Part model, mm, in its own coordinate system. Face numbers are marked on the shaded views. Round coordinates to 2 decimals unless told otherwise and drop trailing zeros. Order: outer loops, then holes, each group sorted by start corner. A loop starts at its lowest first (then second) coordinate and runs counter-clockwise, first axis right, second up. Notation, with made-up numbers: M 28,56 L 60,56 A15 cw 60,77 Z; hole C 25,44.25 d4. An arc over 180 degrees is marked long. One line per question, with ' | ' between items.
from build123d import *

# Parameters (mm, degrees)
F0_R           = 5.5
F1_DEPTH       = 18
F2_R           = 1
F3_R           = 4.375
F4_DEPTH       = 7.5
F5_SIZE        = 1
F7_D           = 5
F7_CSINK_D     = 9
F7_CSINK_ANGLE = 90


with BuildPart() as f1:
    # F0 (on Front) → F1 (new body)
    with BuildSketch(Plane.XZ):
        Circle(F0_R)
    extrude(amount=F1_DEPTH)

    # F2
    f2_edges = [f1.edges().sort_by_distance(p)[0] for p in [
        (-5.5, -18, 0),
    ]]
    fillet(f2_edges, radius=F2_R)

    # F3 (on face) → F4 (join)
    with BuildSketch(Plane(origin=(0, 0, 0), x_dir=(-1, 0, 0), z_dir=(0, 1, 0))):
        Circle(F3_R)
    extrude(amount=F4_DEPTH)

    # F5
    f5_edges = [f1.edges().sort_by_distance(p)[0] for p in [
        (4.375, 7.5, 0),
    ]]
    chamfer(f5_edges, length=F5_SIZE)

    # F7 (through all)
    with Locations(Plane.XZ.offset(18)):
        with Locations((0, 0)):
            CounterSinkHole(F7_D / 2, F7_CSINK_D / 2, counter_sink_angle=F7_CSINK_ANGLE)


solid = f1.part
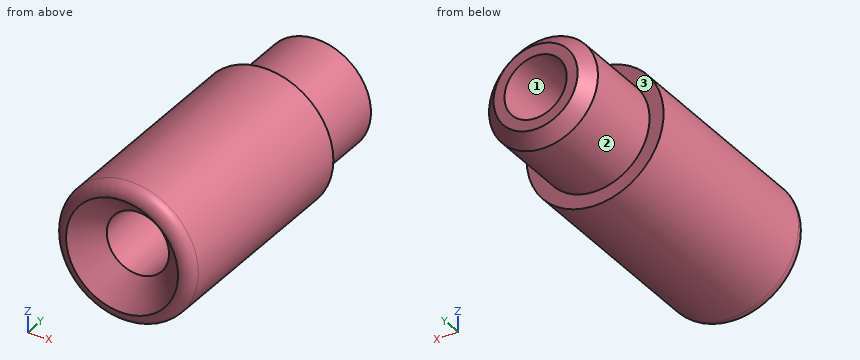
1) Probe line 1 (Z direction, x = 0, y = -4); line 2 (Z direction, x = 0, y = 0.25) (3 decimals); line 3 (X direction, y = -7.25, z = 1). List the from-to ranges inside material, lowest first. Write a range as [from, to].
The answers:
line 1: z = [-5.5, -2.5], [2.5, 5.5] | line 2: z = [-4.375, -2.5], [2.5, 4.375] | line 3: x = [-5.41, -2.29], [2.29, 5.41]
2) Saw through at C-C (y = -8.75). List the corners of the cut face in (x, z).
The answers:
outline: C 0,0 d11; hole C 0,0 d5
3) Saw through at A-A (x = 0). List the corners of the cut face in (y, z) (3 decimals).
The answers:
outline: M -18,-4.5 A1 ccw -17,-5.5 L 0,-5.5 L 0,-4.375 L 6.5,-4.375 L 7.5,-3.375 L 7.5,-2.5 L -16,-2.5 Z; M -18,4.5 L -16,2.5 L 7.5,2.5 L 7.5,3.375 L 6.5,4.375 L 0,4.375 L 0,5.5 L -17,5.5 A1 ccw Z
4) Saw through at B-B (z = 0). List the corners of the cut face in (x, y) (3 decimals), plus the area to 3 significant figures.
The answers:
outline: M -5.5,-17 A1 ccw -4.5,-18 L -2.5,-16 L -2.5,7.5 L -3.375,7.5 L -4.375,6.5 L -4.375,0 L -5.5,0 Z; M 2.5,-16 L 4.5,-18 A1 ccw 5.5,-17 L 5.5,0 L 4.375,0 L 4.375,6.5 L 3.375,7.5 L 2.5,7.5 Z | area: 131 mm²
5) Saw through at D-D (y = 1.75). List the corners of the cut face in (x, z) (3 decimals).
The answers:
outline: C 0,0 d8.75; hole C 0,0 d5
6) Drop flat-ended pins along their axis: pin 1 (2 mm diameter, centred on x = -1, y = 3.5, fed in from +Z) (3 decimals); pin 2 (4 mm diameter, centred on x = -4, y = 0, fed in from +Z). Give the stop position or say it passes through.
The answers:
pin 1: stops at z = 4.375 | pin 2: stops at z = 5.12
7) Two-plate mould, pull along Z, no slides. Class the marked faces 1, 2 and 3: released by +Z, released by -Z, zero draft, split by the parting line, or undercut.
The answers:
face 1: undercut | face 2: split by the parting line | face 3: zero draft
